Can you work these out from the model? Positions are in its coordinate system, mm. Face numbers are marked on the shaded views. Give positions to 0.01 mm unless a question says otherwise; leave off trailing zeros. Order: outer loops, then holes, each group sorted by start corner. A loop starts at its lowest first (then second) coordinate and runs counter-clockwise, first axis right, second up. Notation, with made-up numbers: (0, 37) -> (32, 37) arc R19 cw to (32, 70) -> close; hole circle Ø3 at (-13, 77.25). An arc over 180 degrees is marked (long way). Answer as CSV lines item,"result".
```python
from build123d import *

# Parameters (mm, degrees)
ESBO_O1_W                = 150
ESBO_O1_H                = 100
RESSALTO_EXTRUS_O1_DEPTH = 3
ESBO_O1_3_W              = 135
ESBO_O1_3_H              = 85
ESBO_O1_3_W_2            = 130
ESBO_O1_3_H_2            = 80
RESSALTO_EXTRUS_O2_DEPTH = 6
ESBO_O2_R                = 4
RESSALTO_EXTRUS_O3_DEPTH = 15
ESBO_O3_R                = 1.75
CORTE_EXTRUS_O1_DEPTH    = 8
ESBO_O4_W                = 14
ESBO_O4_H                = 1.980707968
RESSALTO_EXTRUS_O4_DEPTH = 2
ESBO_O5_R                = 11
ESBO_O5_R_2              = 1.5
CORTE_EXTRUS_O2_DEPTH    = 10
CHANFRO1_SIZE            = 2
CHANFRO1_SIZE_2          = 2.965121937
ESBO_O6_W                = 150
ESBO_O6_H                = 100
ESBO_O6_W_2              = 145
ESBO_O6_H_2              = 95
CORTE_EXTRUS_O3_DEPTH    = 10


with BuildPart() as part:
    # Esboço1 → Ressalto-extrusão1 (new body)
    with BuildSketch(Plane.XY):
        with Locations((75, 50)):
            Rectangle(ESBO_O1_W, ESBO_O1_H)
    extrude(amount=RESSALTO_EXTRUS_O1_DEPTH)

    # Esboço1<3> → Ressalto-extrusão2 (add)
    with BuildSketch(Plane.XY):
        with Locations((75, 50)):
            Rectangle(ESBO_O1_3_W, ESBO_O1_3_H)
        with Locations((75, 50)):
            Rectangle(ESBO_O1_3_W_2, ESBO_O1_3_H_2, mode=Mode.SUBTRACT)
    extrude(amount=-RESSALTO_EXTRUS_O2_DEPTH)

    # Esboço2 → Ressalto-extrusão3 (add)
    with BuildSketch(Plane(origin=(0, 0, 0), x_dir=(-1, 0, 0), z_dir=(0, 0, -1))):
        with Locations((-130, 73.25)):
            Circle(ESBO_O2_R)
        with Locations((-32, 76.75)):
            Circle(ESBO_O2_R)
        with Locations((-28, 25.75)):
            Circle(ESBO_O2_R)
        with Locations((-124, 23.25)):
            Circle(ESBO_O2_R)
    extrude(amount=RESSALTO_EXTRUS_O3_DEPTH)

    # Esboço3 → Corte-extrusão1 (cut)
    with BuildSketch(Plane(origin=(0, 0, -15), x_dir=(-1, 0, 0), z_dir=(0, 0, -1))):
        with Locations((-130, 73.25)):
            Circle(ESBO_O3_R)
        with Locations((-32, 76.75)):
            Circle(ESBO_O3_R)
        with Locations((-28, 25.75)):
            Circle(ESBO_O3_R)
        with Locations((-124, 23.25)):
            Circle(ESBO_O3_R)
    extrude(amount=-CORTE_EXTRUS_O1_DEPTH, mode=Mode.SUBTRACT)

    # Esboço4 → Ressalto-extrusão4 (add)
    with BuildSketch(Plane(origin=(0, 0, 0), x_dir=(-1, 0, 0), z_dir=(0, 0, -1))):
        with Locations((-75, 84.770026355)):
            Rectangle(ESBO_O4_W, ESBO_O4_H)
    extrude(amount=RESSALTO_EXTRUS_O4_DEPTH)

    # Esboço5 → Corte-extrusão2 (cut)
    with BuildSketch(Plane(origin=(0, 0, 0), x_dir=(-1, 0, 0), z_dir=(0, 0, -1))):
        with Locations((-75, 50)):
            Circle(ESBO_O5_R)
        with Locations((-85, 60)):
            Circle(ESBO_O5_R_2)
        with Locations((-65, 40)):
            Circle(ESBO_O5_R_2)
        with Locations((-85, 40)):
            Circle(ESBO_O5_R_2)
        with Locations((-65, 60)):
            Circle(ESBO_O5_R_2)
    extrude(amount=-CORTE_EXTRUS_O2_DEPTH, mode=Mode.SUBTRACT)

    # Chanfro1
    # the kernel refuses this chamfer: 2.965121937, 2 mm, written as the material it takes off along each edge
    with BuildSketch(Plane(origin=(75, 50, 0), x_dir=(-1, 0, 0), z_dir=(0, -1, 0))) as chanfro1_piece_1:
        Polygon((11, -CHANFRO1_SIZE), (11 + CHANFRO1_SIZE_2, 0), (11, 0), align=None)
    revolve(axis=Axis((75, 50, 0), (0, 0, -1)), mode=Mode.SUBTRACT)

    # Esboço6 → Corte-extrusão3 (cut)
    with BuildSketch(Plane(origin=(0, 0, 0), x_dir=(-1, 0, 0), z_dir=(0, 0, -1))):
        with Locations((-75, 50)):
            Rectangle(ESBO_O6_W, ESBO_O6_H)
        with Locations((-75, 50)):
            Rectangle(ESBO_O6_W_2, ESBO_O6_H_2, mode=Mode.SUBTRACT)
    extrude(amount=-CORTE_EXTRUS_O3_DEPTH, mode=Mode.SUBTRACT)


solid = part.part
```
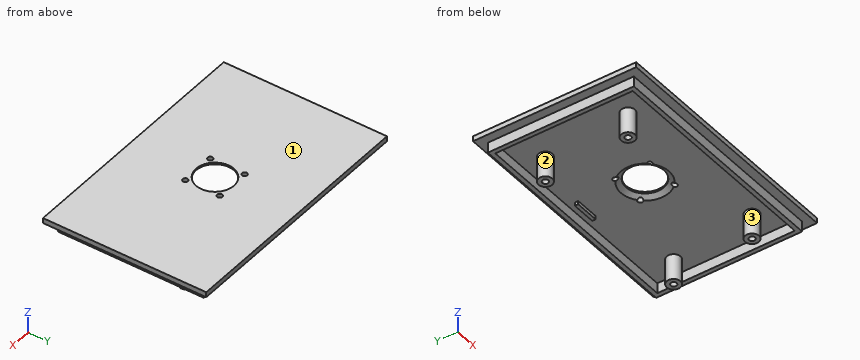
Item 1: Imagine slicing it at A-A, the plane z = -9. Please give me the cut outline in (x, y), then the cut area to 3 significant figures.
Numbers:
outline,"circle Ø8 at (28, 25.75); circle Ø8 at (32, 76.75); circle Ø8 at (124, 23.25); circle Ø8 at (130, 73.25); hole circle Ø3.5 at (28, 25.75); hole circle Ø3.5 at (32, 76.75); hole circle Ø3.5 at (124, 23.25); hole circle Ø3.5 at (130, 73.25)"
area,"163 mm²"
Item 2: Please list where these lines run through material, in increasing order: line 1 along Y through (x, z) = (130, -10); line 2 along Y through (x, z) = (28.5, -7.75); line 3 along X through (y, z) = (60, 0.8).
Numbers:
line 1,"y = 69.25 to 71.5, 75 to 77.25"
line 2,"y = 21.78 to 24.07, 27.43 to 29.72, 74.81 to 78.69"
line 3,"x = 2.5 to 63.5, 66.5 to 67.04, 82.96 to 83.5, 86.5 to 147.5"
Item 3: For pin 1 (1.8 mm diameter, centred on x = 52, z = -3.5, fed in from +Y); pin 2 (1.6 mm diameter, centred on y = 85, z = -1, fed in from -X); pin 3 (1 mm diameter, centred on x = 40, y = 66, fed in from -Z), each with a flat end and sliding along its axis, tell me the tip position at first contact or that it passes through.
Numbers:
pin 1,"stops at y = 92.5"
pin 2,"stops at x = 7.5"
pin 3,"stops at z = 0"
Item 4: Imagine slicing it at C-C, the plane x = 130. Please give me the cut outline in (y, z).
Numbers:
outline,"(2.5, 0) -> (7.5, 0) -> (7.5, -6) -> (10, -6) -> (10, 0) -> (69.25, 0) -> (69.25, -15) -> (71.5, -15) -> (71.5, -7) -> (75, -7) -> (75, -15) -> (77.25, -15) -> (77.25, 0) -> (90, 0) -> (90, -6) -> (92.5, -6) -> (92.5, 0) -> (97.5, 0) -> (97.5, 3) -> (2.5, 3) -> close"
Item 5: We'd pull the mould along X, two halves only. Please class the marked faces 1, 2 and 3: released by +X, released by -X, zero draft, split by the parting line, or undercut.
Numbers:
face 1,"zero draft"
face 2,"undercut"
face 3,"undercut"
Item 6: Imagine slicing it at B-B, the plane x = 40.5. Please give me the cut outline in (y, z), then the cut area to 3 significant figures.
Numbers:
outline,"(2.5, 0) -> (7.5, 0) -> (7.5, -6) -> (10, -6) -> (10, 0) -> (90, 0) -> (90, -6) -> (92.5, -6) -> (92.5, 0) -> (97.5, 0) -> (97.5, 3) -> (2.5, 3) -> close"
area,"315 mm²"
